Autodesk Inventor part; units mm, degrees
ref_plane "YZ Plane" through (0, 0, 0) normal (1, 0, 0) x (0, 1, 0)
ref_plane "XZ Plane" through (0, 0, 0) normal (0, 1, 0) x (-1, 0, 0)
ref_plane "XY Plane" through (0, 0, 0) normal (0, 0, 1) x (1, 0, 0)
sketch "Sketch1" plane through (0, 0, 0) normal (0, 0, 1) x (1, 0, 0)
  line L0 (-0.7938, 0) -> (4.7625, 0)
  line L1 (0, -20.5581) -> (0, 20.5581)
  line L2 (3.9688, 12.7) -> (3.9688, -12.7)
  arc A0 (3.9688, 12.7) -> (0, 12.7) centre (1.9844, 12.7) ccw
  arc A1 (0, -12.7) -> (3.9688, -12.7) centre (1.9844, -12.7) ccw
  arc A2 (0.7938, -12.7) -> (3.175, -12.7) centre (1.9844, -12.7) ccw
  line L3 (3.175, -12.7) -> (3.175, 12.7)
  arc A3 (3.175, 12.7) -> (0.7938, 12.7) centre (1.9844, 12.7) ccw
  line L4 (0, 12.7) -> (0.7938, 12.7)
  line L5 (0.7938, -12.7) -> (0, -12.7)
  line L6 (0, -12.7) -> (0, 12.7) construction
  point P0 (0, 0)
  point P1 (3.9688, 0)
  dimension "d0" = 0.7937
  dimension "d1" = 3.9688
  dimension "d2" = 25.4
extrude "Extrusion1" add sketch "Sketch1" along normal mid plane 457.2 contours L3 A3 L4 A0 L2 L0 | L0 L2 A1 L5 A2 L3
properties part number "slide outer" material "Steel"
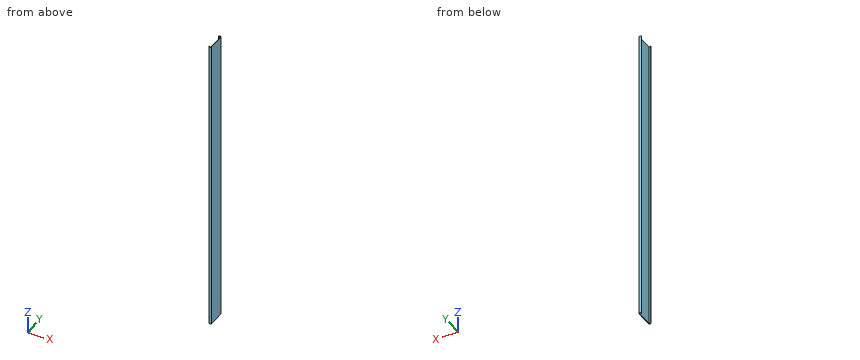
Work out the finished part from the listing and answer in its coordinate system (mm). Give positions to 0.01 mm unless a question says otherwise; leave off trailing zeros. Loops run counter-clockwise (first coordinate to the right, second up) from the corner with the lowest first, then second, coordinate; pieces in that order, holes last. Notation, with made-up numbers: (-20, 52) -> (19, 52) arc R9 ccw to (19, 65) -> close; hole circle Ø3 at (22, -2). An arc over 180 degrees is marked (long way). Use CSV: the item, a comma, the result in double quotes.
1. Straight lines are drawn through the part: line 1 (Y direction, x = 1.85, z = -47); line 2 (Y direction, x = 0.35, z = -29); line 3 (X direction, y = 1.75, z = -77) (3 decimals). For each, find the intervals that lie inside material, in ascending order.
Found:
line 1,"-14.68 to -13.88, 13.88 to 14.68"
line 2,"-13.83 to -12.7, 12.7 to 13.83"
line 3,"3.175 to 3.969"
2. A flat-ended cylindrical pin translates along its axis: pin 1 Ø5 at (y, z) = (-2, -133.5) entering from -X (3 decimals). Find the tip coordinate at first contact, or state that the pin passes through.
Found:
pin 1,"x = 3.175"
3. The part is cut by section C-C (y = -7.5). Write down the section's boundary in (x, z) (3 decimals).
Found:
outline,"(3.175, -228.6) -> (3.969, -228.6) -> (3.969, 228.6) -> (3.175, 228.6) -> close"
4. The part is cut by section A-A (x = 1.9). Write down the section's boundary in (y, z).
Found:
outline,"(-14.68, -228.6) -> (-13.89, -228.6) -> (-13.89, 228.6) -> (-14.68, 228.6) -> close; (13.89, -228.6) -> (14.68, -228.6) -> (14.68, 228.6) -> (13.89, 228.6) -> close"
